Work out the finished part from the listing and answer in its coordinate system (mm). Face numbers are marked on the shaded views. A direction names the side the tool comes from. Give positions to 0.01 mm unless a question says otherwise; leave off trailing zeros. Loops run counter-clockwise (first coordinate to the right, second up) from the corner with the lowest first, then second, coordinate; pieces in that order, holes last. Notation, with made-up numbers: (-0.75, 74.25) - (49.25, 74.25) arc R21 ccw to (49.25, 95.25) - close; hole circle Ø4 at (29, 48.25). An arc over 180 degrees is marked (long way). Use one line per item in the form item = value. Start each with the question number.
from build123d import *

# Parameters (mm, degrees)
F0_R      = 19.05
F0_R_2    = 12.7
F1_DEPTH  = 25.4
F2_R      = 31.75
F3_DEPTH  = 25.4
F3_FACE_R = 12.7
F4_DEPTH  = 25.4


with BuildPart() as f1:
    # F0 (on Right) → F1 (new body)
    with BuildSketch(Plane.YZ):
        Circle(F0_R)
        Circle(F0_R_2, mode=Mode.SUBTRACT)
    extrude(amount=-F1_DEPTH)

    # F2 (on Right) → F3 (join)
    with BuildSketch(Plane.YZ):
        Circle(F2_R)
    extrude(amount=F3_DEPTH)

    # F3_face (on face) → F4 (cut)
    with BuildSketch(Plane(origin=(0, 0, 0), x_dir=(0, 1, 0), z_dir=(-1, 0, 0))):
        Circle(F3_FACE_R)
    extrude(amount=-F4_DEPTH, mode=Mode.SUBTRACT)


solid = f1.part
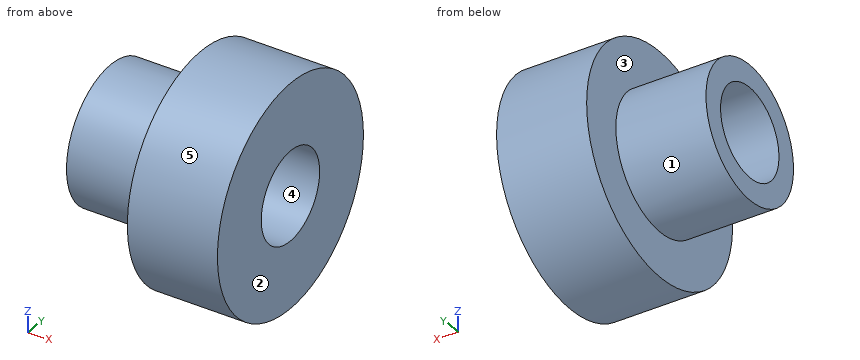
1) Flat-ended cylindrical pins translate along their axes: pin 1 Ø8 at (x, y) = (17, 1.5) entering from -Z; pin 2 Ø10 at (x, y) = (17, -7.5) entering from -Z; pin 3 Ø5 at (x, z) = (-2, 9) entering from -Y; pin 4 Ø10 at (y, z) = (22, -6.5) entering from -X. Find the tip coordinate at first contact, or state that the pin passes through.
2) A cutting plane is placed at D-D (y = -23). Give the vertices of the cut face in (x, z), plus the area to 3 significant figures.
3) A cutting plane is placed at C-C (x = -3.5). Give the vertices of the cut face in (y, z), plus the area to 3 significant figures.
4) Determine the mould class of the marked faces 3, 4 and 5 for opening direction Y: released by +Y, released by -Y, zero draft, split by the parting line, or undercut.
5) Find the intervals of material crossed by probe 1 along Z at (x, y) = (-10, -0.5); probe 2 along Z at (x, y) = (10, 0); probe 3 along X at (y, z) = (29.5, -1), in increasing order.
6) A cutting plane is placed at A-A (z = 0). Give the vertices of the cut face in (x, y).
7) A tool of negligible diameter and unlimited length cuts with its end or side. For the marked faces 1 and 2, from which of +Z, -Z, +X, -X, +Y, -Y can it reach the whole face along a straight path? Write none if from no direction.
Answer sheet:
q1.pin_1 = -31.75
q1.pin_2 = -31.65
q1.pin_3 = -30.85
q1.pin_4 = -25.4
q2.outline = (0, -21.89) - (25.4, -21.89) - (25.4, 21.89) - (0, 21.89) - close
q2.area = 1,110 mm²
q3.outline = circle Ø38.1 at (0, 0); hole circle Ø25.4 at (0, 0)
q3.area = 633 mm²
q4.face_3 = zero draft
q4.face_4 = undercut
q4.face_5 = split by the parting line
q5.probe_1 = -19.04 to -12.69, 12.69 to 19.04
q5.probe_2 = -31.75 to -12.7, 12.7 to 31.75
q5.probe_3 = 0 to 25.4
q6.outline = (-25.4, -19.05) - (0, -19.05) - (0, -31.75) - (25.4, -31.75) - (25.4, -12.7) - (-25.4, -12.7) - close; (-25.4, 12.7) - (25.4, 12.7) - (25.4, 31.75) - (0, 31.75) - (0, 19.05) - (-25.4, 19.05) - close
q7.face_1 = -X
q7.face_2 = +Z, -Z, +X, +Y, -Y
